Can you work these out from the model? Positions are in its coordinate system, mm. Round coordinates to 2 decimals unless told otherwise and drop trailing zeros. Write each loop counter-clockwise with the first axis right and the second up, starting at its lowest first coordinate (ties: lowest second). Pieces come first, ordered by that corner, then holes. Notation, with made-up numbers: (-33, 6.5) -> (-18, 6.5) arc R18 cw to (-18, 16.5) -> close; hole circle Ø10 at (15, -31). An arc over 180 degrees is marked (long way). Write item = value, one per line. Start each with the question number.
1) Imagine slicing it at A-A, the plane z = 2.25. Please give me the cut outline in (x, y).
2) If I drill on line 1 (Y direction, x = 0, z = 4.5); line 2 (Y direction, x = 0.3, z = -3.5); line 3 (X direction, y = 0.2, z = 2), over which ranges is the centre line in solid material (lowest first)?
3) Thinking about a two-plate mould opening in X: for faces 1 (the face through (0, 0, 10)), 2 (the face through (-0.57, -0.18, -2.78)), which applies, +X half, -X half, draft (parallel to the pull), parting line (faces both ways), or undercut?
Autodesk Inventor part; units mm, degrees
ref_plane "YZ Plane" through (0, 0, 0) normal (1, 0, 0) x (0, 1, 0)
ref_plane "XZ Plane" through (0, 0, 0) normal (0, 1, 0) x (-1, 0, 0)
ref_plane "XY Plane" through (0, 0, 0) normal (0, 0, 1) x (1, 0, 0)
sketch "Sketch1" plane through (0, 0, 0) normal (0, 1, 0) x (-1, 0, 0)
  line L0 (1, 0) -> (0.1812, -5.6471)
  line L1 (1, 0) -> (0.75, 0)
  line L2 (0.75, 0) -> (0.75, 10)
  line L3 (0.75, 10) -> (0, 10)
  line L4 (0, 10) -> (0, -5.8903)
  arc A0 (0, -6.8827) -> (0.002, -6.8828) centre (0.001, -6.8827) ccw
  arc A1 (0.0897, -5.8553) -> (0.1812, -5.6471) centre (-0.2406, -5.586) ccw
  arc A2 (0, -5.8903) -> (0.1211, -5.8114) centre (0.0001, -5.7581) ccw
  point P0 (0, 0)
  dimension "d7" = 0.25
  dimension "d9" = 0.001
revolve "Revolution1" add sketch "Sketch1" angle 360 about axis through (0, 0, 10) along (0, 0, -1)
properties part number "Pencil Tip"
Reported:
q1.outline = circle Ø1.5 at (0, 0)
q2.line_1 = -0.75 to 0.75
q2.line_2 = -0.39 to 0.39
q2.line_3 = -0.72 to 0.72
q3.face_1 = draft
q3.face_2 = parting line
